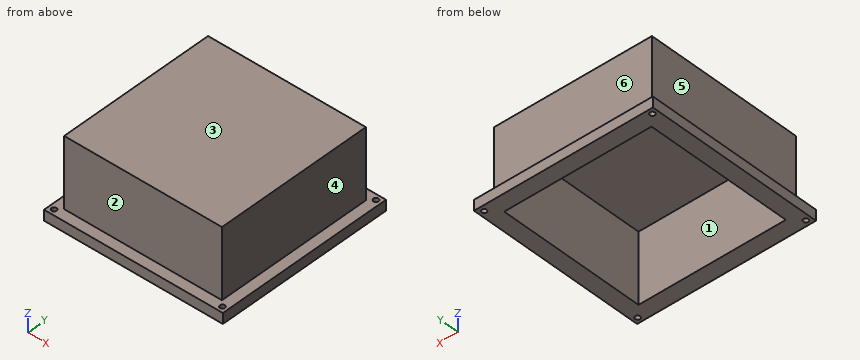
```python
from build123d import *

# Parameters (mm, degrees)
SKETCH6_W           = 95.25
SKETCH6_H           = 95.25
SKETCH6_W_2         = 88.9
SKETCH6_H_2         = 88.9
BOSS_EXTRUDE3_DEPTH = 42.164
SKETCH7_W           = 107.95
SKETCH7_H           = 107.95
SKETCH7_R           = 1.5
SKETCH7_W_2         = 95.25
SKETCH7_H_2         = 95.25
BOSS_EXTRUDE4_DEPTH = 6.35
SKETCH8_W           = 95.25
SKETCH8_H           = 95.25
BOSS_EXTRUDE5_DEPTH = 6.35


with BuildPart() as part:
    # Sketch6 → Boss-Extrude3 (new body)
    with BuildSketch(Plane.XY):
        Rectangle(SKETCH6_W, SKETCH6_H)
        Rectangle(SKETCH6_W_2, SKETCH6_H_2, mode=Mode.SUBTRACT)
    extrude(amount=BOSS_EXTRUDE3_DEPTH)

    # Sketch7 → Boss-Extrude4 (add)
    with BuildSketch(Plane.XY):
        Rectangle(SKETCH7_W, SKETCH7_H)
        with Locations((-50.8, 50.8)):
            Circle(SKETCH7_R, mode=Mode.SUBTRACT)
        with Locations((50.8, 50.8)):
            Circle(SKETCH7_R, mode=Mode.SUBTRACT)
        with Locations((-50.8, -50.8)):
            Circle(SKETCH7_R, mode=Mode.SUBTRACT)
        with Locations((50.8, -50.8)):
            Circle(SKETCH7_R, mode=Mode.SUBTRACT)
        Rectangle(SKETCH7_W_2, SKETCH7_H_2, mode=Mode.SUBTRACT)
    extrude(amount=BOSS_EXTRUDE4_DEPTH)

    # Sketch8 → Boss-Extrude5 (add)
    with BuildSketch(Plane.XY.offset(42.164)):
        Rectangle(SKETCH8_W, SKETCH8_H)
    extrude(amount=BOSS_EXTRUDE5_DEPTH)


solid = part.part
```
Check sheet for the modelled part. Datum: model origin and axes. Units: mm. Face numbers are marked on the shaded views. A direction names the side the tool comes from. Give positions to 0.01 mm unless a question says otherwise; leave off trailing zeros. Order: outer loops, then holes, each group sorted by start corner. A loop starts at its lowest first (then second) coordinate and runs counter-clockwise, first axis right, second up. Notation, with made-up numbers: (27.25, 74.5) -> (31.25, 74.5) arc R31 ccw to (31.25, 113.5) -> close; hole circle Ø7 at (87.5, 33.25). An arc over 180 degrees is marked (long way). Use CSV: the item, a comma, the result in double quotes. Start each with the question number.
1) Sectioned sample at A-A, the plane x = -50.8. Record the boundary of the cut face in (y, z) (3 decimals).
2) Go/stop test with flat-tipped pins: P1, Ø8, axis at x = -18.5, z = 24, coming from the +Y side (3 decimals); P2, Ø4, axis at x = -50.8, y = 50.8, coming from the +Z side; P3, Ø2, axis at y = 13.5, z = 16.5, coming from the -X side (3 decimals). Record where each tip stops, or that it passes through.
3) Mould release check, pull along Y, two halves, no side actions. Record for the marked faces 1, 2 and 3: released by +Y, released by -Y, zero draft, split by the parting line, or undercut.
4) Set-up check for the marked faces 4, 5 and 6: record each of +Z, -Z, +X, -X, +Y, -Y from which the full face is reachable in a straight line by a thin tool's end or side.
5) Sectioned sample at C-C, the plane z = 29. Record the boundary of the cut face in (x, y) (3 decimals), plus the area to 3 significant figures.
6) Sectioned sample at D-D, the plane x = -6.5. Record the boundary of the cut face in (y, z) (3 decimals), plus the area to 3 significant figures.
7) Material ranges on line 1 (Y direction, x = 50.8, z = 2.5) (3 decimals); line 2 (Y direction, x = -42, z = 42) (3 decimals), recorded low to high. Write a range as from..to.
Recorded:
1,outline,"(-53.975, 0) -> (-52.3, 0) -> (-52.3, 6.35) -> (-53.975, 6.35) -> close; (-49.3, 0) -> (49.3, 0) -> (49.3, 6.35) -> (-49.3, 6.35) -> close; (52.3, 0) -> (53.975, 0) -> (53.975, 6.35) -> (52.3, 6.35) -> close"
2,P1,"y = 47.625"
2,P2,"z = 6.35"
2,P3,"x = -47.625"
3,face 1,"undercut"
3,face 2,"released by -Y"
3,face 3,"zero draft"
4,face 4,"+Z, +X, +Y, -Y"
4,face 5,"+Z, -X, +Y, -Y"
4,face 6,"+Z, +X, -X, +Y"
5,outline,"(-47.625, -47.625) -> (47.625, -47.625) -> (47.625, 47.625) -> (-47.625, 47.625) -> close; hole (-44.45, -44.45) -> (44.45, -44.45) -> (44.45, 44.45) -> (-44.45, 44.45) -> close"
5,area,"1,170 mm2"
6,outline,"(-53.975, 0) -> (-44.45, 0) -> (-44.45, 42.164) -> (44.45, 42.164) -> (44.45, 0) -> (53.975, 0) -> (53.975, 6.35) -> (47.625, 6.35) -> (47.625, 48.514) -> (-47.625, 48.514) -> (-47.625, 6.35) -> (-53.975, 6.35) -> close"
6,area,"953 mm2"
7,line 1,"-53.975..-52.3, -49.3..49.3, 52.3..53.975"
7,line 2,"-47.625..-44.45, 44.45..47.625"
